The listing builds one solid part. Answer for the finished solid, in the listing's coordinates (mm). A direction names the side the tool comes from. Round coordinates to 2 decimals unless told otherwise and drop trailing zeros. Write each loop counter-clockwise with the first axis right and the second up, starting at its lowest first coordinate (ties: lowest second). Pieces come first, ordered by that corner, then holes.
from build123d import *

# Parameters (mm, degrees)
F0_W           = 50.8
F0_H           = 127
F1_DEPTH       = 10
F2_R           = 5.08
F4_D           = 7
F6_D           = 6.6
F6_CBORE_D     = 11.25
F6_CBORE_DEPTH = 6


with BuildPart() as f1:
    # F0 (on Front) → F1 (new body)
    with BuildSketch(Plane.XZ):
        Rectangle(F0_W, F0_H)
    extrude(amount=F1_DEPTH)

    # F2
    f2_edges = [f1.edges().sort_by_distance(p)[0] for p in [
        (25.4, -5, 63.5),
        (25.4, -5, -63.5),
        (-25.4, -5, -63.5),
        (-25.4, -5, 63.5),
    ]]
    fillet(f2_edges, radius=F2_R)

    # F4 (through all)
    with Locations(Plane.XZ.offset(10)):
        with Locations((0, 48.26), (0, -48.26)):
            Hole(F4_D / 2)

    # F6 (through all)
    with Locations(Plane.XZ.offset(10)):
        with Locations((-18.122286547, 17.5), (16.877713453, 17.5), (16.877713453, -17.5), (-18.122286547, -17.5)):
            CounterBoreHole(F6_D / 2, F6_CBORE_D / 2, F6_CBORE_DEPTH)


solid = f1.part
1. Given pin 1 (4 mm diameter, centred on x = 0, z = -48.26, fed in from +Y); pin 2 (3.5 mm diameter, centred on x = 17.5, z = 19.5, fed in from -Y); pin 3 (14.5 mm diameter, centred on x = -18.12, z = 17.5, fed in from -Y), each flat-ended and moving along its own axis, determine where each tip first touches the part or whether it passes through.
Geometry says:
pin 1: passes through
pin 2: stops at y = -4
pin 3: stops at y = -10
2. Section C-C on z = -17.5 is taken. Determine the outline of the cut face in (x, y), plus the area to 3 significant figures.
Geometry says:
outline: (-25.4, -10) - (-23.75, -10) - (-23.75, -4) - (-21.42, -4) - (-21.42, 0) - (-25.4, 0) - close; (-14.82, -4) - (-12.5, -4) - (-12.5, -10) - (11.25, -10) - (11.25, -4) - (13.58, -4) - (13.58, 0) - (-14.82, 0) - close; (20.18, -4) - (22.5, -4) - (22.5, -10) - (25.4, -10) - (25.4, 0) - (20.18, 0) - close
area: 320 mm2
3. Section A-A on x = 0 is taken. Determine the outline of the cut face in (y, z), plus the area to 3 significant figures.
Geometry says:
outline: (-10, -63.5) - (0, -63.5) - (0, -51.76) - (-10, -51.76) - close; (-10, -44.76) - (0, -44.76) - (0, 44.76) - (-10, 44.76) - close; (-10, 51.76) - (0, 51.76) - (0, 63.5) - (-10, 63.5) - close
area: 1,130 mm2
4. A tool of negligible diameter and unlimited length cuts with its end or side. For faces 4 (the face through (-23.951, -5.07, -61.972)), 5 (the face through (17, -4, -21)), from which of +Z, -Z, +X, -X, +Y, -Y can it reach the whole face along a straight path? Write none if from no direction.
Geometry says:
face 4: -Z, -X, +Y, -Y
face 5: -Y
5. For a pull along X with two mould halves and no side action, classify faces 1 (the face through (23.872, -5.07, -62.051)), 2 (the face through (17, -4, 14)), 3 (the face through (0, -5, -63.5)) as released by +X, released by -X, zero draft, split by the parting line, or undercut.
Geometry says:
face 1: released by +X
face 2: undercut
face 3: zero draft
6. Straight lines are drawn through the part: line 1 along Z through (x, y) = (19.5, -3.5); line 2 along Z through (x, y) = (19, -5.25); line 3 along Y through (x, z) = (-21.5, -17). For each, find the intervals that lie inside material, in ascending order.
Geometry says:
line 1: z = -63.5 to -19.5, -15.5 to 15.5, 19.5 to 63.5
line 2: z = -63.5 to -22.71, -12.29 to 12.29, 22.71 to 63.5
line 3: y = -4 to 0
7. Section B-B on y = -5.25 is taken. Determine the outline of the cut face in (x, z) (3 decimals), plus the area to 3 significant figures.
Geometry says:
outline: (-25.4, -58.42) arc R5.08 ccw to (-20.32, -63.5) - (20.32, -63.5) arc R5.08 ccw to (25.4, -58.42) - (25.4, 58.42) arc R5.08 ccw to (20.32, 63.5) - (-20.32, 63.5) arc R5.08 ccw to (-25.4, 58.42) - close; hole circle Ø11.25 at (-18.122, -17.5); hole circle Ø11.25 at (-18.122, 17.5); hole circle Ø7 at (0, -48.26); hole circle Ø7 at (0, 48.26); hole circle Ø11.25 at (16.878, -17.5); hole circle Ø11.25 at (16.878, 17.5)
area: 5,950 mm2
8. Section D-D on z = -48.26 is taken. Determine the outline of the cut face in (x, y).
Geometry says:
outline: (-25.4, -10) - (-3.5, -10) - (-3.5, 0) - (-25.4, 0) - close; (3.5, -10) - (25.4, -10) - (25.4, 0) - (3.5, 0) - close
